Autodesk Inventor part; units mm, degrees
ref_plane "YZ Plane" through (0, 0, 0) normal (1, 0, 0) x (0, 1, 0)
ref_plane "XZ Plane" through (0, 0, 0) normal (0, 1, 0) x (-1, 0, 0)
ref_plane "XY Plane" through (0, 0, 0) normal (0, 0, 1) x (1, 0, 0)
sketch "Sketch2" plane through (0, 0, 0) normal (0, 1, 0) x (-1, 0, 0)
  line L0 (450, 0) -> (139.0576, -427.9754) construction
  line L1 (139.0576, -427.9754) -> (-364.0576, -264.5034) construction
  line L2 (-364.0576, -264.5034) -> (-364.0576, 264.5034) construction
  line L3 (-364.0576, 264.5034) -> (139.0576, 427.9754) construction
  line L4 (139.0576, 427.9754) -> (450, 0) construction
  circle A0 centre (0, 0) radius 450 construction
  line L5 (-250, 0) -> (-77.2542, 237.7641) construction
  line L6 (-77.2542, 237.7641) -> (202.2542, 146.9463) construction
  line L7 (202.2542, 146.9463) -> (202.2542, -146.9463) construction
  line L8 (202.2542, -146.9463) -> (-77.2542, -237.7641) construction
  line L9 (-77.2542, -237.7641) -> (-250, 0) construction
  circle A1 centre (0, 0) radius 250 construction
  line L10 (450, 0) -> (202.2542, 146.9463)
  line L11 (139.0576, 427.9754) -> (202.2542, 146.9463)
  line L12 (139.0576, 427.9754) -> (-77.2542, 237.7641)
  line L13 (-77.2542, 237.7641) -> (-364.0576, 264.5034)
  line L14 (-250, 0) -> (-364.0576, 264.5034)
  line L15 (-250, 0) -> (-364.0576, -264.5034)
  line L16 (-77.2542, -237.7641) -> (-364.0576, -264.5034)
  line L17 (202.2542, -146.9463) -> (139.0576, -427.9754)
  line L18 (-77.2542, -237.7641) -> (139.0576, -427.9754)
  line L19 (450, 0) -> (202.2542, -146.9463)
  dimension "d17" = 500
  dimension "d16" = 450
extrude "Extrusion2" add sketch "Sketch2" along normal mid plane 100
fillet "Fillet1" radius 50 1 edges at (-139.0576, 0, 427.9754)
fillet "Fillet2" radius 50 9 edges at (364.0576, 0, 264.5034) (364.0576, 0, -264.5034) (-139.0576, 0, -427.9754) (-450, 0, 0) (-202.2542, 0, -146.9463) (-202.2542, 0, 146.9463) (77.2542, 0, -237.7641) (250, 0, 0) (77.2542, 0, 237.7641)
properties part number "star"
Model file for the job. Use its own axes, mm. A direction names the side the tool comes from. Give positions to 0.01 mm unless a question says otherwise; leave off trailing zeros. Loops run counter-clockwise (first coordinate to the right, second up) from the corner with the lowest first, then second, coordinate; pieces in that order, holes last. Notation, with made-up numbers: (37, 88.5) -> (91, 88.5) arc R29 ccw to (91, 111.5) -> close; hole circle Ø7 at (8.25, -39). An arc over 180 degrees is marked (long way). Write each question's results on one line, items separated by ' | '.
(1) Probe line 1 along Z through (x, y) = (262.5, 31.5); line 2 along Z through (x, y) = (274.5, 16); line 3 along Z through (x, y) = (-326, 10). List the from-to ranges inside material, lowest first.
Geometry results:
line 1: z = -255.03 to -28.99, 28.99 to 255.03 | line 2: z = -256.15 to -56.82, 56.82 to 256.15 | line 3: z = -73.55 to 73.55
(2) Cut at A-A on y = -38.5. List the corners of the cut face in (x, z), and give its area (3 significant figures).
Geometry results:
outline: (-377.5, -43) -> (-220.8, -135.95) arc R50 cw to (-197.52, -167.98) -> (-157.55, -345.73) arc R50 ccw to (-75.75, -372.31) -> (61.06, -252) arc R50 cw to (98.72, -239.77) -> (280.12, -256.68) arc R50 ccw to (330.68, -187.1) -> (258.54, -19.8) arc R50 cw to (258.54, 19.8) -> (330.68, 187.1) arc R50 ccw to (280.12, 256.68) -> (98.72, 239.77) arc R50 cw to (61.06, 252) -> (-75.75, 372.31) arc R50 ccw to (-157.55, 345.73) -> (-197.52, 167.98) arc R50 cw to (-220.8, 135.95) -> (-377.5, 43) arc R50 ccw to start | area: 323,000 mm²
(3) Flat gauge pins, fed straight in: pin 1 Ø3 at (x, y) = (-277.5, 15) entering from +Z; pin 2 Ø2 at (x, y) = (54.5, 30) entering from +Z; pin 3 Ø12 at (y, z) = (12.5, 58.5) entering from -X. Where does each tip first touch, or does it go through?
Geometry results:
pin 1: stops at z = 103.21 | pin 2: stops at z = 258.65 | pin 3: stops at x = -361.49
(4) Tool access for faces 1 (the flat face through (-300.244, -0.7, 88.825)), 2 (the flat face through (294.103, -0.7, -102.276)): list every direction of +Z, -Z, +X, -X, +Y, -Y with a clear straight run to the whole face (end or side of a thin tool).
Geometry results:
face 1: +Z, -X, +Y, -Y | face 2: +X, +Y, -Y
(5) Cut at C-C on z = 97. List the corners of the cut face in (x, y).
Geometry results:
outline: (-286.46, -50) -> (291.83, -50) -> (291.83, 50) -> (-286.46, 50) -> close
(6) Cut at B-B on x = 73. List the corners of the cut face in (y, z).
Geometry results:
outline: (-50, -244.21) -> (50, -244.21) -> (50, 244.21) -> (-50, 244.21) -> close
(7) Pull direction Z, two halves, no side cores. Call faces 3 (the cylindrical face through (-124.909, -0.7, -382.085)), 4 (the flat face through (188.153, -0.7, 248.103)), 5 (the cylindrical face through (254.45, -0.7, 0.28)): released by +Z, released by -Z, zero draft, split by the parting line, or undercut.
Geometry results:
face 3: released by -Z | face 4: released by +Z | face 5: undercut
